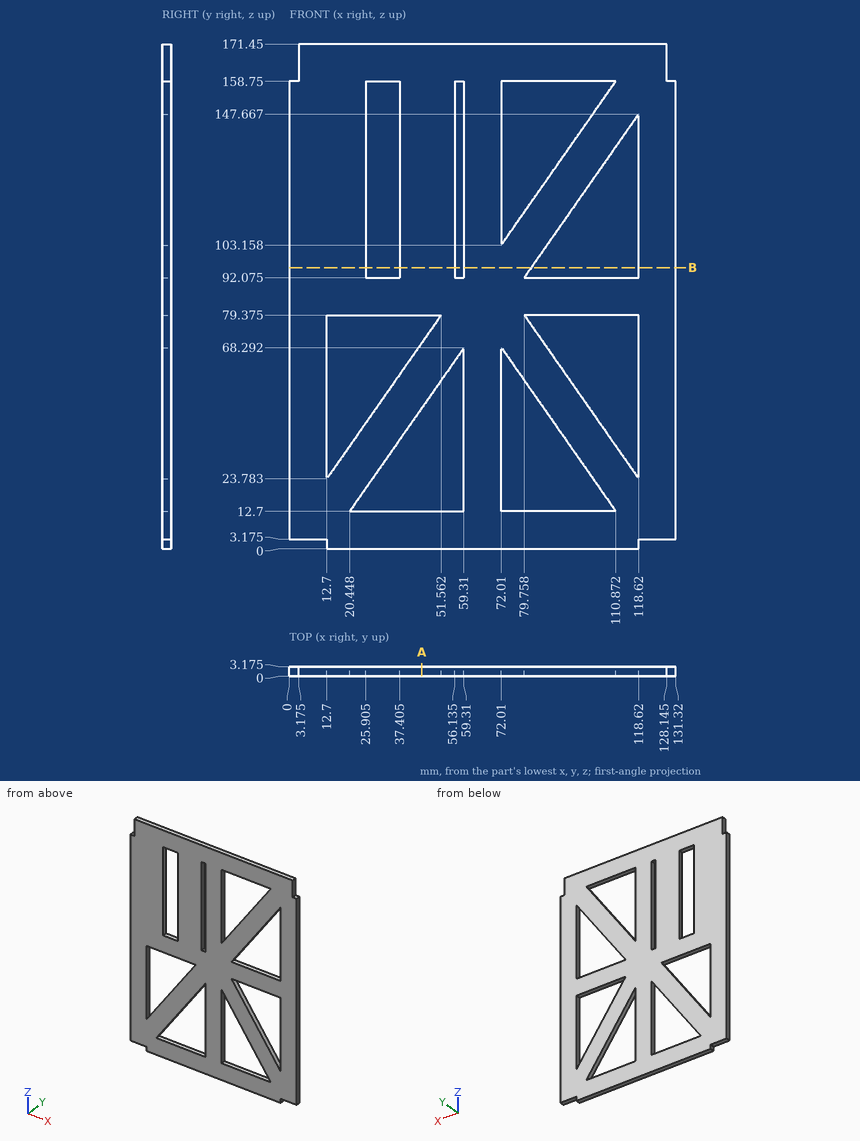
Drawing for the job (mm, zero at the part's lowest x, y, z). Coordinates: 2 decimals unless noted, no trailing zeros. Order: outer loops, then holes, each group sorted by start corner. A loop starts at its lowest first (then second) coordinate and runs counter-clockwise, first axis right, second up. Notation, with made-up numbers: (70, 15.5) -> (107, 15.5) arc R9 ccw to (107, 31.5) -> close; hole circle Ø3 at (69, 9). An arc over 180 degrees is marked (long way). Return JSON: item names as keys, results as strings.
Item 1: Slice it at B-B (z = 95.5). Write the cut outline in (x, y) (1 decimal).
Model answer:
{"outline": "(0, 0) -> (25.9, 0) -> (25.9, 3.2) -> (0, 3.2) -> close; (37.4, 0) -> (56.1, 0) -> (56.1, 3.2) -> (37.4, 3.2) -> close; (59.3, 0) -> (82.2, 0) -> (82.2, 3.2) -> (59.3, 3.2) -> close; (118.6, 0) -> (131.3, 0) -> (131.3, 3.2) -> (118.6, 3.2) -> close"}
Item 2: Slice it at A-A (x = 45). Count the separate pieces of the cut face and the enclosed holes in it, then the cut area to 3 significant figures.
Model answer:
{"separate pieces": "3", "enclosed holes": "0", "area": "403 mm²"}
Item 3: Pin check, flat tip, straight feed: P1, Ø1, axis at y = 1.5, z = 2, coming from the +X side. Stop position of the tip, or through.
Model answer:
{"P1": "stops at x = 118.62"}
Item 4: Wall check: line 1 along X through (y, z) = (1.65, 55) (1 decimal); line 2 along X through (y, z) = (2.5, 127.5) (1 decimal); line 3 along X through (y, z) = (1.2, 77.5). Give the ranges that are in metal, low to high. Write a range as from..to.
Model answer:
{"line 1": "x = 0..12.7, 34.5..50, 59.3..72, 81.3..96.8, 118.6..131.3", "line 2": "x = 0..25.9, 37.4..56.1, 59.3..72, 89..104.5, 118.6..131.3", "line 3": "x = 0..12.7, 50.25..81.07, 118.62..131.32"}
